Here's the drawing with two shaded views (mm, measured from the low corner). I have some questions. Coordinates: 2 decimals unless noted, no trailing zeros. Loops run counter-clockwise (first coordinate to the right, second up) from the corner with the lowest first, then second, coordinate; pieces in that order, holes last. Notation, with made-up numbers: (-11.5, -16.5) -> (15.5, -16.5) arc R32 ccw to (15.5, 12.5) -> close; hole circle Ø1 at (-25.75, 72). An arc over 180 degrees is marked (long way). Answer as a JSON object with one key per item and string values. Group by question number.
1) I need wall thicknesses on probe 1 along Z at (x, y) = (68.5, 1.1) (1 decimal); probe 2 along X at (y, z) = (2.2, 131.5). Which ranges of each line are inside material? Lowest first, please. Write a range as [from, to].
2) I want a section at A-A (z = 67.5). Count the separate pieces of the cut face and the enclosed holes in it.
3) I want a section at B-B (x = 81.5). Write out the boundary of the cut face in (y, z) (1 decimal).
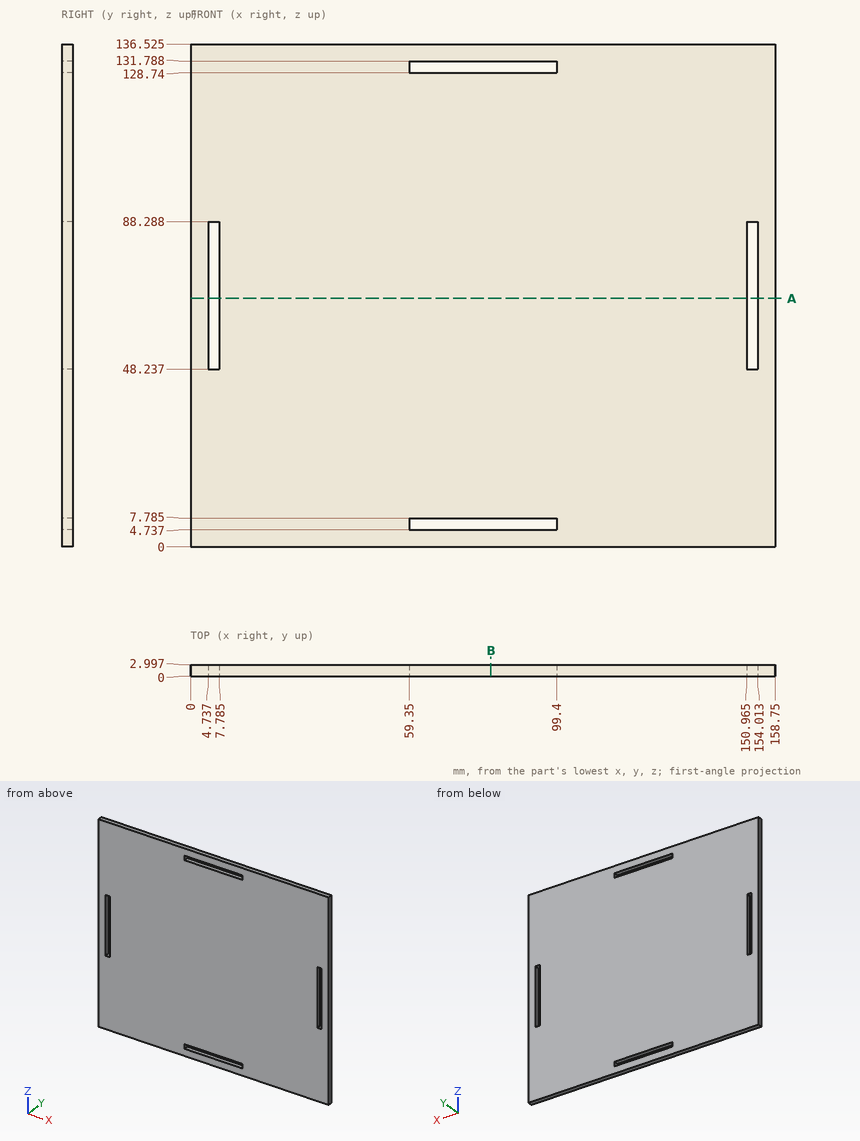
Determined:
{
 "1": {"probe 1": "[0, 4.7], [7.8, 128.7], [131.8, 136.5]", "probe 2": "[0, 59.35], [99.4, 158.75]"},
 "2": {"separate pieces": "3", "enclosed holes": "0"},
 "3": {"outline": "(0, 0) -> (3, 0) -> (3, 4.7) -> (0, 4.7) -> close; (0, 7.8) -> (3, 7.8) -> (3, 128.7) -> (0, 128.7) -> close; (0, 131.8) -> (3, 131.8) -> (3, 136.5) -> (0, 136.5) -> close"}
}
